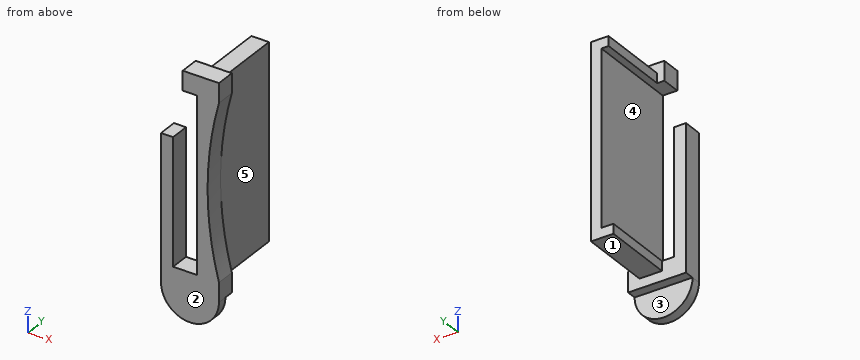
Autodesk Inventor part; units mm, degrees
ref_plane "YZ Plane" through (0, 0, 0) normal (1, 0, 0) x (0, 1, 0)
ref_plane "XZ Plane" through (0, 0, 0) normal (0, 1, 0) x (-1, 0, 0)
ref_plane "XY Plane" through (0, 0, 0) normal (0, 0, 1) x (1, 0, 0)
sketch "Sketch1" plane through (0, 0, 0) normal (0, 1, 0) x (-1, 0, 0)
  line L0 (0, 0) -> (0, -36)
  line L1 (0, -36) -> (5, -36)
  line L2 (7.5, -40) -> (-4.5, -40)
  line L3 (-4.5, -40) -> (-4.5, -36)
  arc A0 (-4.5, -36) -> (-4.5, 0) centre (-72.1461, -18) ccw
  line L4 (-4.5, 0) -> (-4.5, 4)
  line L5 (-4.5, 4) -> (3, 4)
  line L6 (3, 4) -> (3, 0)
  line L7 (3, 0) -> (0, 0)
  line L8 (7.5, -40) -> (7.5, -10)
  line L9 (7.5, -10) -> (5, -10)
  line L10 (5, -10) -> (5, -36)
  dimension "d0" = 36
  dimension "d1" = 5
  dimension "d4" = 12
  dimension "d6" = 70
  dimension "d7" = 4
  dimension "d8" = 7.5
  dimension "d20" = 30
extrude "Extrusion1" add sketch "Sketch1" along normal blind 4
sketch "Sketch2" plane through (0, 0, 0) normal (0, -1, 0) x (1, 0, 0)
  line L0 (-7.5, -40) -> (4.5, -40)
  arc A0 (-7.5, -40) -> (4.5, -40) centre (-1.5, -40) ccw
  line L1 (4.5, -40) -> (-7.5, -40)
  point P0 (0, 0)
extrude "Extrusion2" add sketch "Sketch2" against normal blind 2
sketch "Sketch3" plane through (0, 4, 0) normal (0, 1, 0) x (1, 0, 0)
  line L0 (0, 0) -> (-1.5, 0)
  line L1 (-3, 0) -> (0, 0)
  line L2 (-1.5, 0) -> (-1.5, -2)
  arc A0 (4.5, 36) -> (4.5, 0) centre (72.1461, 18) ccw
  line L3 (2.1461, 18) -> (2.1461, -2)
  line L4 (2.1461, -2) -> (-1.5, -2)
  line L5 (0, 36) -> (-5, 36)
  line L6 (-2.5, 36) -> (-2.5, 38)
  line L7 (2.1461, 18) -> (2.1461, 38)
  line L8 (2.1461, 38) -> (-2.5, 38)
  line L9 (0, 36) -> (0, 0)
  line L10 (0, 0) -> (0, 36)
  line L11 (0, 36) -> (-2.5, 36)
  dimension "d15" = 2
  dimension "d17" = 2
extrude "Extrusion3" add sketch "Sketch3" along normal blind 15
properties part number "sem2_plateclip"
The model under review builds one solid part; all positions refer to its coordinate system, in mm. Face numbers are marked on the shaded views. A direction names the side the tool comes from. Coordinates: 2 decimals unless noted, no trailing zeros. Write each loop counter-clockwise with the first axis right and the second up, starting at its lowest first coordinate (ties: lowest second). Pieces come first, ordered by that corner, then holes.
1) Machinability: for the marked faces 1 and 2, which of the approach directions +Z, -Z, +X, -X, +Y, -Y give a long, thin tool a straight path to every point of the face, cutting with its end or side? Answer none if there is none.
2) We need section D-D on z = -0.5. State the section outline as (x, y) points, then the cut area to 3 significant figures.
3) We need section B-B on y = 17.5. State the section outline as (x, z) points, then the cut area to 3 significant figures.
4) Clearance check with flat-ended pins moving along their axes: pin 1 Ø5 at (x, y) = (-1, 11) entering from -Z; pin 2 Ø3 at (x, y) = (-6, 1) entering from +Z; pin 3 Ø3 at (x, z) = (-4, -43) entering from +Y. State where each tip first meets the part, or that it passes through.
5) The part is to be moulded in two halves that separate along X. For the marked faces 3, 4 and 5, say which applies: pulls with the +X half, pulls with the -X half, needs draft (parallel to the pull), parting line crosses it, or undercut.
6) We need section C-C on x = -1. State the section outline as (y, z) points.
7) To check wall thickness, follow probe 1 along Z at (x, y) = (-0.5, 7.75); probe 2 along Y at (x, z) = (-1.5, -39.5); probe 3 along Z at (x, y) = (0.25, 15). State the ranges of each line that lie inside material, in increasing order.
8) We need section A-A on z = -33. State the section outline as (x, y) points.
Answer list:
1. face 1: -Z, +X, -X, +Y
1. face 2: +Z, -Z, +X, -X, -Y
2. outline: (0, 0) - (4.37, 0) - (4.37, 4) - (2.15, 4) - (2.15, 19) - (0, 19) - close
2. area: 49.7 mm2
3. outline: (-2.5, -38) - (2.15, -38) - (2.15, 2) - (-1.5, 2) - (-1.5, 0) - (0, 0) - (0, -36) - (-2.5, -36) - close
3. area: 93.8 mm2
4. pin 1: stops at z = -38
4. pin 2: stops at z = -10
4. pin 3: stops at y = 2
5. face 3: needs draft
5. face 4: undercut
5. face 5: pulls with the +X half
6. outline: (0, -45.98) - (2, -45.98) - (2, -40) - (4, -40) - (4, -38) - (19, -38) - (19, -36) - (0, -36) - close; (0, 0) - (19, 0) - (19, 2) - (4, 2) - (4, 4) - (0, 4) - close
7. probe 1: z = -38 to -36, 0 to 2
7. probe 2: y = 0 to 4
7. probe 3: z = -38 to 2
8. outline: (-7.5, 0) - (-5, 0) - (-5, 4) - (-7.5, 4) - close; (0, 0) - (3.77, 0) - (3.77, 4) - (2.15, 4) - (2.15, 19) - (0, 19) - close
